Drawing for the job (mm, zero at the part's lowest x, y, z). Give positions to 0.01 mm unless a question says otherwise; leave off trailing zeros. Write each loop counter-clockwise with the first axis right and the second up, starting at its lowest first coordinate (ties: lowest second). Pieces come first, ordered by that corner, then holes. Notation, with made-up numbers: M 47,72 L 74,72 A28 cw 74,98 Z; hole C -12,-9 d9. An arc over 180 degrees is marked long. Use CSV: the item, a comma, the result in double quotes. Start each with the question number.
1. Band-saw the part on C-C, the plane x = 4. List the corners of the cut face in (y, z).
2. Band-saw the part on A-A, the plane z = 2.5. List the corners of the cut face in (x, y), then the cut area to 3 significant figures.
3. Drop flat-ended pins along their axis: pin 1 Ø0.6 at (x, z) = (0, 2) entering from -Y; pin 2 Ø1.8 at (y, z) = (1.58, 2.5) entering from -X. Give the stop position or say it passes through.
4. Band-saw the part on B-B, the plane y = 1.58. List the corners of the cut face in (x, z).
5. Mould opens along Z. For the marked faces 1, 2 and 3 say: pulls with the +Z half, pulls with the -Z half, needs draft (parallel to the pull), parting line crosses it, or undercut.
6. Drill centre lines: line 1 along Y through (x, z) = (4.9, 2.5); line 2 along X through (y, z) = (0.2, 4.55); line 3 along Y through (x, z) = (4.25, 2.25). Where is each one in solid material? Low to high. Write a range as from..to.
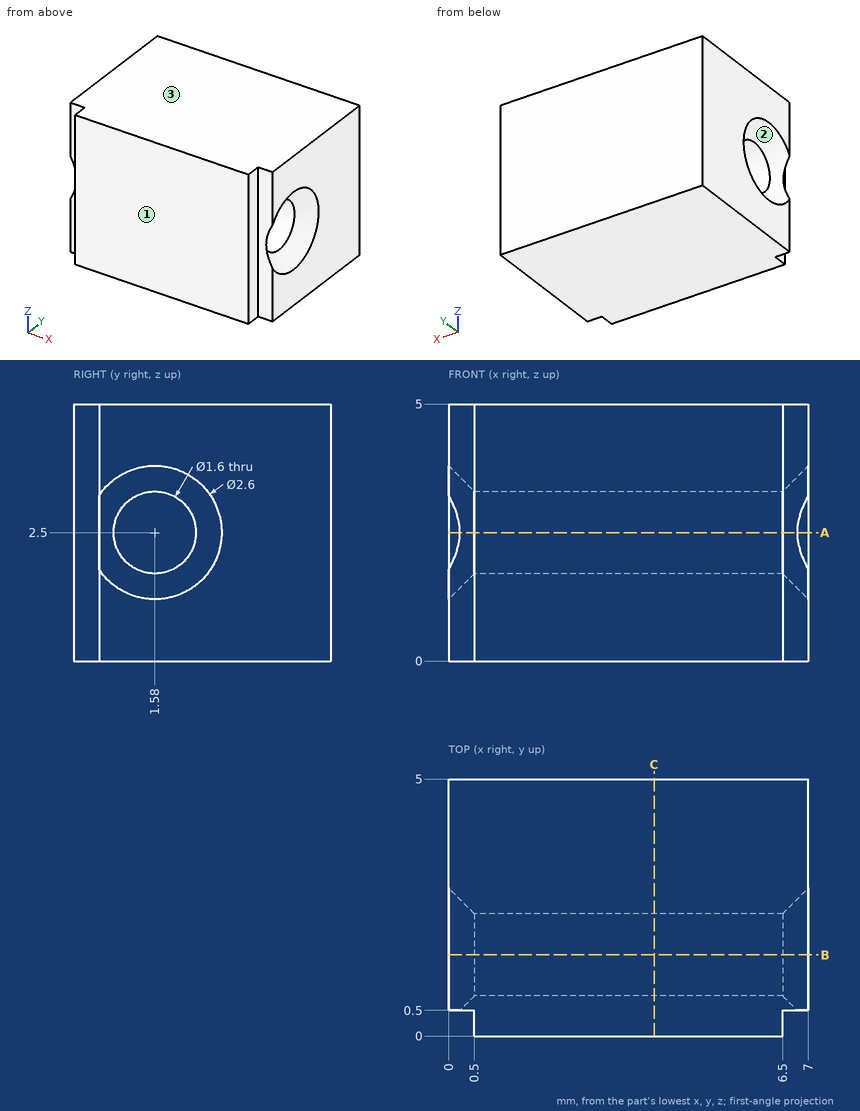
Output:
1,outline,"M 0,0 L 5,0 L 5,5 L 0,5 Z; hole C 1.58,2.5 d1.6"
2,outline,"M 0,2.88 L 0.5,2.38 L 6.5,2.38 L 7,2.88 L 7,5 L 0,5 Z; M 0.22,0.5 L 0.5,0.5 L 0.5,0 L 6.5,0 L 6.5,0.5 L 6.78,0.5 L 6.5,0.78 L 0.5,0.78 Z"
2,area,"22.8 mm²"
3,pin 1,"stops at y = 0.5"
3,pin 2,"stops at x = 0.4"
4,outline,"M 0,0 L 7,0 L 7,1.2 L 6.5,1.7 L 0.5,1.7 L 0,1.2 Z; M 0,3.8 L 0.5,3.3 L 6.5,3.3 L 7,3.8 L 7,5 L 0,5 Z"
5,face 1,"needs draft"
5,face 2,"undercut"
5,face 3,"pulls with the +Z half"
6,line 1,"y = 0..0.78, 2.38..5"
6,line 2,"x = 0.5..6.5"
6,line 3,"y = 0..0.82, 2.34..5"
